```python
from build123d import *

# Parameters (mm, degrees)
SKETCH_2_R               = 51.1
SKETCH_2_R_2             = 49.5
EXTRUDE_1_DEPTH          = 15
SKETCH_3_R               = 2.1
CUT_EXTRUDE_1_DEPTH      = 60
CUT_EXTRUDE_START        = -15
CUT_EXTRUDE_2_DEPTH      = 15
PATTERN_CIRCULAR_4_COUNT = 6
PATTERN_CIRCULAR_5_COUNT = 6
CHAMFER_1_SIZE           = 1


with BuildPart() as part:
    # Эскиз2 → Бобышка-Вытянуть1 (new body)
    with BuildSketch(Plane(origin=(0, 0, 0), x_dir=(1, 0, 0), z_dir=(0, 1, 0))):
        with Locations(Location((0, 0, 0), (0, 0, 270))):
            Circle(SKETCH_2_R)
        with Locations(Location((0, 0, 0), (0, 0, 270))):
            Circle(SKETCH_2_R_2, mode=Mode.SUBTRACT)
    extrude(amount=EXTRUDE_1_DEPTH)

    # Эскиз3 → Вырез-Вытянуть1 (cut)
    with BuildSketch(Plane.XY):
        with Locations(Location((0, 7.5, 0), (0, 0, 90))):
            Circle(SKETCH_3_R)
    cut_extrude_1 = extrude(amount=-CUT_EXTRUDE_1_DEPTH, mode=Mode.SUBTRACT)

    # Эскиз5 → Вырез-Вытянуть2 (cut)
    with BuildSketch(Plane(origin=(0, 15, 0), x_dir=(1, 0, 0), z_dir=(0, 1, 0)).offset(CUT_EXTRUDE_START)):
        with BuildLine():
            Line((-4.5, -50.901473456), (4.5, -50.901473456))
            ThreePointArc((4.5, -50.901473456), (0, -51.1), (-4.5, -50.901473456))
        make_face()
    cut_extrude_2 = extrude(amount=CUT_EXTRUDE_2_DEPTH, mode=Mode.SUBTRACT)

    # Круговой массив4: Вырез-Вытянуть2 ×6 about axis
    pattern_circular_4_axis = Axis((0, 0, 0), (0, 1, 0))
    for i in range(1, PATTERN_CIRCULAR_4_COUNT):
        add(cut_extrude_2.rotate(pattern_circular_4_axis, i * 360 / PATTERN_CIRCULAR_4_COUNT), mode=Mode.SUBTRACT)

    # Круговой массив5: Вырез-Вытянуть1 ×6 about axis
    pattern_circular_5_axis = Axis((0, 15, 0), (0, 1, 0))
    for i in range(1, PATTERN_CIRCULAR_5_COUNT):
        add(cut_extrude_1.rotate(pattern_circular_5_axis, i * 360 / PATTERN_CIRCULAR_5_COUNT), mode=Mode.SUBTRACT)

    # Фаска1
    chamfer_1_edges = [part.edges().sort_by_distance(p)[0] for p in [
        (0, 5.4, -50.901473456),
        (0, 5.4, 50.901473456),
        (44.081969103, 5.4, 25.450736728),
        (44.081969103, 5.4, -25.450736728),
        (-44.081969103, 5.4, -25.450736728),
        (-44.081969103, 5.4, 25.450736728),
    ]]
    chamfer(chamfer_1_edges, length=CHAMFER_1_SIZE)


solid = part.part
```
Here's how the part is built. I have some questions about the finished solid (model axes, mm). Give positions to 0.01 mm unless a question says otherwise; leave off trailing zeros. Loops run counter-clockwise (first coordinate to the right, second up) from the corner with the lowest first, then second, coordinate; pieces in that order, holes last. Notation, with made-up numbers: M 68,8.5 L 119,8.5 A15 cw 119,14.5 Z; hole C -6,66.5 d3. An arc over 180 degrees is marked long. Put each result on its own line as item: value. Start each with the question number.
(1) I want a section at A-A on x = 0. Please give me the cut outline in (y, z), then the cut area to 3 significant figures.
(2) I need wall thicknesses on line 1 along Y through (x, z) = (0, 49.7); line 2 along X through (y, z) = (11, 0.5); line 3 along Z through (x, y) = (0, 3). Which ranges of each line are inside material? Lowest first, please. Write a range as [from, to].
(3) I want a section at C-C on y = 12.5. Please give me the cut outline in (x, z).
(4) If we mould it in two halves opening along Y, with no side actions, what happens to faces 1 (the flat face through (44.11, 4.06, -25.4)), 2 (the flat face through (-11, 0, 49)), 3 (the cylindrical face through (-0.8, 9.44, 49.68))? For each: +Y half, -Y half, draft (parallel to the pull), parting line (faces both ways), or undercut.
(5) Will these pins go through, and if not, where does the flat tip stop? pin 1 Ø1 at (x, y) = (34.5, 13.5) entering from +Z; pin 2 Ø4 at (x, y) = (23, 10) entering from -Z; pin 3 Ø5 at (x, y) = (0, 7.5) entering from -Z.
(6) I want a section at B-B on z = 0. Please give me the cut outline in (x, y).
(7) I want a section at D-D on x = 11.5. Please give me the cut outline in (y, z).
Answer block:
1. outline: M 0,-50.9 L 4.4,-50.9 L 5.4,-49.9 L 5.4,-49.5 L 0,-49.5 Z; M 0,49.5 L 5.4,49.5 L 5.4,49.9 L 4.4,50.9 L 0,50.9 Z; M 9.6,-49.9 L 10.6,-50.9 L 15,-50.9 L 15,-49.5 L 9.6,-49.5 Z; M 9.6,49.5 L 15,49.5 L 15,50.9 L 10.6,50.9 L 9.6,49.9 Z
1. area: 28.3 mm^2
2. line 1: [0, 5.4], [9.6, 15]
2. line 2: [-51.1, -49.5], [49.5, 51.1]
2. line 3: [-50.9, -49.5], [49.5, 50.9]
3. outline: M -46.33,-21.55 L -41.83,-29.35 A51.1 ccw -4.5,-50.9 L 4.5,-50.9 A51.1 ccw 41.83,-29.35 L 46.33,-21.55 A51.1 ccw 46.33,21.55 L 41.83,29.35 A51.1 ccw 4.5,50.9 L -4.5,50.9 A51.1 ccw -41.83,29.35 L -46.33,21.55 A51.1 ccw Z; hole C 0,0 d99
4. face 1: draft
4. face 2: -Y half
4. face 3: undercut
5. pin 1: z = 38.15
5. pin 2: z = -46.59
5. pin 3: z = -50.3
6. outline: M -51.1,0 L -49.5,0 L -49.5,15 L -51.1,15 Z; M 49.5,0 L 51.1,0 L 51.1,15 L 49.5,15 Z
7. outline: M 0,-49.79 L 15,-49.79 L 15,-48.15 L 0,-48.15 Z; M 0,48.15 L 15,48.15 L 15,49.79 L 0,49.79 Z
